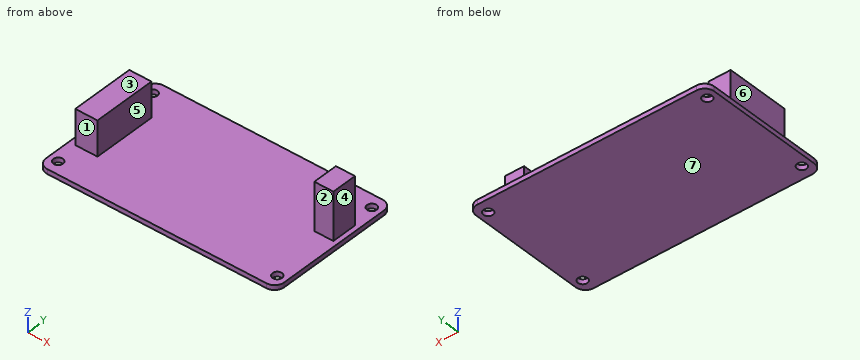
```python
from build123d import *

# Parameters (mm, degrees)
F0_W     = 75
F0_H     = 43
F1_DEPTH = 1.5
F3_D     = 3
F4_R     = 3
F5_W     = 7
F5_H     = 20
F6_DEPTH = 11
F7_W     = 6
F7_H     = 8
F8_DEPTH = 15


with BuildPart() as f1:
    # F0 (on Top) → F1 (new body)
    with BuildSketch(Plane.XY):
        Rectangle(F0_W, F0_H)
    extrude(amount=F1_DEPTH)

    # F3 (through all)
    with Locations(Plane.XY.offset(1.5)):
        with Locations((-34.5, 17.5), (34.5, 17.5), (34.5, -17.5), (-34.5, -17.5)):
            Hole(F3_D / 2)

    # F4
    f4_edges = [f1.edges().sort_by_distance(p)[0] for p in [
        (-37.5, -21.5, 0.75),
        (37.5, -21.5, 0.75),
        (-37.5, 21.5, 0.75),
        (37.5, 21.5, 0.75),
    ]]
    fillet(f4_edges, radius=F4_R)

    # F5 (on face) → F6 (join)
    with BuildSketch(Plane.XY.offset(1.5)):
        with Locations((-32, 0)):
            Rectangle(F5_W, F5_H)
    extrude(amount=F6_DEPTH)

    # F7 (on face) → F8 (join)
    with BuildSketch(Plane.XY.offset(1.5)):
        with Locations((33, 5.5)):
            Rectangle(F7_W, F7_H)
    extrude(amount=F8_DEPTH)


solid = f1.part
```
Geometry check sheet. Reference: the model listing, model coordinates, mm. Face numbers are marked on the shaded views. A direction names the side the tool comes from. Round coordinates to 2 decimals unless told otherwise and drop trailing zeros. Loops run counter-clockwise (first coordinate to the right, second up) from the corner with the lowest first, then second, coordinate; pieces in that order, holes last. Notation, with made-up numbers: (31, 57) - (83, 57) arc R37 ccw to (83, 95) - close; hole circle Ø11 at (33.25, 9). An arc over 180 degrees is marked (long way). Write each question's results on one line, items separated by ' | '. Start each with the question number.
Q1. Access from +Z, -Z, +X, -X, +Y, -Y to the whole of each face (thin tool, end or side, straight path). Record for the marked faces 1, 2, 3 and 4.
Q2. Cross-section at C-C on x = 32. Enter the section's corners in (y, z), and give its area (4 significant figures).
Q3. Gauge pin test, flat ends, axial feed: P1, Ø1, axis at y = -4, z = 5, coming from the +X side; P2, Ø6.5, axis at y = 6.5, z = 8, coming from the +X side; P3, Ø4, axis at y = 4.5, z = 12.5, coming from the -X side. Record the tip position at first contact, or that the pin passes through.
Q4. Cross-section at A-A on y = 17.5. Enter the section's corners in (x, z), and give its area (4 significant figures).
Q5. Release check for a two-part mould opening along X. For the marked faces 5, 6 and 7 record: +X half, -X half, draft (parallel to the pull), parting line (faces both ways), or undercut.
Q6. Cross-section at D-D on y = -11.5. Enter the section's corners in (x, z), and give its area (4 significant figures).
Q7. Cross-section at B-B on z = 6.5. Enter the section's corners in (x, y), and give its area (3 significant figures).
Q8. Thickness scan on line 1 (Y direction, x = 34.5, z = 1.1); line 2 (X direction, y = 7.5, z = 11.25); line 3 (Z direction, x = -1, y = -16). Record the ranges inside material, lowest first. Write a range as [from, to].
Answers below:
1) face 1: +Z, +X, -X, -Y | face 2: +Z, +X, -Y | face 3: +Z, -X, +Y, -Y | face 4: +Z, +X, +Y, -Y
2) outline: (-21.5, 0) - (21.5, 0) - (21.5, 1.5) - (9.5, 1.5) - (9.5, 16.5) - (1.5, 16.5) - (1.5, 1.5) - (-21.5, 1.5) - close | area: 184.5 mm²
3) P1: stops at x = -28.5 | P2: stops at x = 36 | P3: stops at x = -35.5
4) outline: (-37.5, 0) - (-36, 0) - (-36, 1.5) - (-37.5, 1.5) - close; (-33, 0) - (33, 0) - (33, 1.5) - (-33, 1.5) - close; (36, 0) - (37.5, 0) - (37.5, 1.5) - (36, 1.5) - close | area: 103.5 mm²
5) face 5: undercut | face 6: -X half | face 7: draft
6) outline: (-37.5, 0) - (37.5, 0) - (37.5, 1.5) - (-37.5, 1.5) - close | area: 112.5 mm²
7) outline: (-35.5, -10) - (-28.5, -10) - (-28.5, 10) - (-35.5, 10) - close; (30, 1.5) - (36, 1.5) - (36, 9.5) - (30, 9.5) - close | area: 188 mm²
8) line 1: y = [-21.5, -19], [-16, 16], [19, 21.5] | line 2: x = [-35.5, -28.5], [30, 36] | line 3: z = [0, 1.5]
